Geometry: final body of the model. Coordinates: model frame, mm. Round coordinates to 2 decimals unless told otherwise and drop trailing zeros. Loops run counter-clockwise (first coordinate to the right, second up) from the corner with the lowest first, then second, coordinate; pieces in that order, holes last. Notation, with made-up numbers: (-16.5, -27) - (12.5, -27) arc R4 ccw to (12.5, -21) - close; hole circle Ø4 at (78, 38). An arc over 180 degrees is marked (long way). Write item = value, one per line. Start each with the question number.
Item 1: Draft query along Y for faces 1 (the cylindrical face through (10.382, -19.961, 32.045)), 2 (the flat face through (-5, -18, 65)), 3 (the cylindrical face through (-4.01, -18.06, 54.15)). Return one class per face: pulls with the +Y half, pulls with the -Y half, needs draft (parallel to the pull), parting line crosses it, or undercut.
Item 2: First-contact query: pin 1 (2 mm diameter, centred on y = 10, z = 7, fed in from -X); pin 2 (8 mm diameter, centred on x = -18, z = 51, fed in from -Y); pin 3 (3 mm diameter, centred on x = -18, z = 14.5, fed in from +Y). Flat tips, straight axial feed; report the tip coordinate or a pass-through.
Item 3: Section D-D (y = 19.5). Return loops of the section in (x, z), plus the area to 3 significant figures.
Item 4: Section C-C (z = 44). Return loops of the section in (x, y), plus the area to 3 significant figures.
Item 5: Section A-A (x = 0). Return loops of the section in (y, z).
Item 6: Line query: line 1 (Y direction, x = 0, z = 19.5); line 2 (Y direction, x = 5, z = 44); line 3 (X direction, y = -5, z = 15). Output: solid intervals per line, ascending. Write a range as from..to.
from build123d import *

# Parameters (mm, degrees)
SKETCH_R        = 22.5
PAD_DEPTH       = 65
SKETCH001_R     = 18.5
POCKET_DEPTH    = 22
SKETCH002_R     = 15.75
POCKET001_DEPTH = 43
CHAMFER_ANGLE   = 12.5
CHAMFER_SIZE    = 12


with BuildPart() as part:
    # Sketch → Pad (new body)
    with BuildSketch(Plane.XY):
        Circle(SKETCH_R)
    extrude(amount=PAD_DEPTH)

    # Sketch001 → Pocket (cut)
    with BuildSketch(Plane.XY.offset(65)):
        Circle(SKETCH001_R)
    extrude(amount=-POCKET_DEPTH, mode=Mode.SUBTRACT)

    # Sketch002 → Pocket001 (cut)
    with BuildSketch(Plane.XY):
        Circle(SKETCH002_R)
    extrude(amount=POCKET001_DEPTH, mode=Mode.SUBTRACT)

    # Chamfer
    chamfer_edges = [part.edges().sort_by_distance(p)[0] for p in [
        (-15.75, 0, 43),
    ]]
    chamfer_side = part.faces().sort_by_distance((-15.75, 0, 21.5))[0]
    chamfer(chamfer_edges, length=CHAMFER_SIZE, angle=CHAMFER_ANGLE, reference=chamfer_side)


solid = part.part
Taken from the geometry:
q1.face_1 = parting line crosses it
q1.face_2 = needs draft
q1.face_3 = undercut
q2.pin_1 = -20.62
q2.pin_2 = -17.61
q2.pin_3 = 15.3
q3.outline = (-11.22, 0) - (11.22, 0) - (11.22, 65) - (-11.22, 65) - close
q3.area = 1,460 mm^2
q4.outline = circle Ø45 at (0, 0); hole circle Ø37 at (0, 0)
q4.area = 515 mm^2
q5.outline = (-22.5, 0) - (-15.75, 0) - (-15.75, 31) - (-18.41, 43) - (-18.5, 43) - (-18.5, 65) - (-22.5, 65) - close; (15.75, 0) - (22.5, 0) - (22.5, 65) - (18.5, 65) - (18.5, 43) - (18.41, 43) - (15.75, 31) - close
q6.line_1 = -22.5..-15.75, 15.75..22.5
q6.line_2 = -21.94..-17.81, 17.81..21.94
q6.line_3 = -21.94..-14.94, 14.94..21.94
